from build123d import *

# Parameters (mm, degrees)
PAD027_DEPTH    = 4
SKETCH057_R     = 1.25
POCKET019_DEPTH = 12.901
FILLET_R        = 3


with BuildPart() as part:
    # Sketch055 → Pad027 (new body, symmetric)
    with BuildSketch(Plane.YZ.offset(-96)):
        Polygon((101, 27.1), (93, 27.1), (93, 32), (101, 40), align=None)
    extrude(amount=PAD027_DEPTH, both=True)

    # Sketch057 (on Face1 of Pad027) → Pocket019 (cut, through all)
    with BuildSketch(Plane.YX.offset(-27.1)):
        with Locations((97, -96)):
            Circle(SKETCH057_R)
    extrude(amount=-POCKET019_DEPTH, mode=Mode.SUBTRACT)

    # Fillet
    fillet_edges = [part.edges().sort_by_distance(p)[0] for p in [
        (-100, 93, 29.55),
        (-100, 97, 36),
        (-92, 97, 36),
        (-92, 93, 29.55),
    ]]
    fillet(fillet_edges, radius=FILLET_R)


with BuildPart() as part_1:
    # Body039 placement: moved
    add(part.part.moved(Location((192, 0, 0))))


solid = part_1.part
Read the model definition and answer for the solid it produces. Units are mm, in the model's axes. Round coordinates to 2 decimals unless told otherwise and drop trailing zeros. Write each loop counter-clockwise with the first axis right and the second up, starting at its lowest first coordinate (ties: lowest second). Pieces come first, ordered by that corner, then holes. Notation, with made-up numbers: (83, 89.25) - (92, 89.25) arc R26 ccw to (92, 120.25) - close; hole circle Ø7 at (44.25, 71.25). An arc over 180 degrees is marked (long way). One line per question, with ' | ' between items. Start each with the question number.
1. Each of these flat-tipped pins is pushed along its axis until it touches: pin 1 (2 mm diameter, centred on x = 94.5, z = 36.5, fed in from -Y); pin 2 (1 mm diameter, centred on x = 95, y = 97, fed in from +Z); pin 3 (4 mm diameter, centred on y = 94.5, z = 36.5, fed in from -X); pin 4 (3 mm diameter, centred on x = 96, y = 97, fed in from +Z). Where does it stop, or does it pass through?
2. Section B-B (x = 96) is taken. Determine the outline of the cut face in (y, z), and give its area (4 significant figures).
3. Find the intervals of material crossed by probe 1 along Y at (x, z) = (96, 29.75); probe 2 along Y at (x, z) = (96.25, 32.5); probe 3 along X at (y, z) = (97, 35), in increasing order. Write a range as [from, to].
4. Section A-A (z = 28.5) is taken. Determine the outline of the cut face in (x, y).
5. For a pull along X with two mould halves and no side action, classify faces 1 (the face through (100, 99, 31)), 2 (the face through (96.38, 98.19, 32.1)), 3 (the face through (96, 101, 34)) as +X half, -X half, draft (parallel to the pull), parting line (faces both ways), or undercut.
Filled in:
1) pin 1: y = 96.53 | pin 2: z = 36.47 | pin 3: through | pin 4: z = 37.5
2) outline: (93, 27.1) - (95.75, 27.1) - (95.75, 34.75) - (93, 32) - close; (98.25, 27.1) - (101, 27.1) - (101, 40) - (98.25, 37.25) - close | area: 48.95 mm²
3) probe 1: [93, 95.75], [98.25, 101] | probe 2: [93.5, 95.78], [98.22, 101] | probe 3: [93.06, 94.75], [97.25, 98.94]
4) outline: (92, 96) arc R3 ccw to (95, 93) - (97, 93) arc R3 ccw to (100, 96) - (100, 101) - (92, 101) - close; hole circle Ø2.5 at (96, 97)
5) face 1: +X half | face 2: undercut | face 3: draft
